```python
from build123d import *

# Parameters (mm, degrees)
F0_R     = 5
F1_DEPTH = 9
F2_R     = 3.5
F3_DEPTH = 8
F4_W     = 9.3990088471
F4_H     = 6
F5_DEPTH = 12.5
F7_DEPTH = 25
F8_R     = 1
F9_DEPTH = 8


with BuildPart() as f1:
    # F0 (on Front) → F1 (new body)
    with BuildSketch(Plane.XZ):
        Circle(F0_R)
    extrude(amount=F1_DEPTH)

    # F2 (on face) → F3 (join)
    with BuildSketch(Plane.XZ.offset(9)):
        Circle(F2_R)
    extrude(amount=F3_DEPTH)

    # F4 (on Right) → F5 (cut, symmetric)
    with BuildSketch(Plane.YZ):
        with Locations((-3.8004955764, 3)):
            Rectangle(F4_W, F4_H)
    extrude(amount=F5_DEPTH, both=True, mode=Mode.SUBTRACT)

    # F6 (on face) → F7 (cut)
    with BuildSketch(Plane(origin=(0, -8.5, 0), x_dir=(-1, 0, 0), z_dir=(0, 1, 0))):
        with BuildLine():
            Line((-1, 3), (1, 3))
            Line((1, 3), (1, 4.8989794856))
            ThreePointArc((1, 4.8989794856), (0, 5), (-1, 4.8989794856))
            Line((-1, 4.8989794856), (-1, 3))
        make_face()
    extrude(amount=-F7_DEPTH, mode=Mode.SUBTRACT)

    # F8 (on face) → F9 (join)
    with BuildSketch(Plane.XY):
        with Locations((0, -4)):
            Circle(F8_R)
    extrude(amount=F9_DEPTH)


solid = f1.part
```
Work out the finished part from the listing and answer in its coordinate system (mm). A direction names the side the tool comes from. Coordinates: 2 decimals unless noted, no trailing zeros. Loops run counter-clockwise (first coordinate to the right, second up) from the corner with the lowest first, then second, coordinate; pieces in that order, holes last. Notation, with made-up numbers: M 24.5,77.5 L 34.5,77.5 A22 cw 34.5,91.5 Z; hole C -27.5,68 d2. An arc over 180 degrees is marked long. Use CSV: the item, a comma, the result in double quotes. Start each with the question number.
(1) Find section C-C, the plane z = -1.75. Give the vertices of the cut face in (x, y), then the cut area to 3 significant figures.
(2) For faces 1 (the face through (-1, -11.79, 3.17)), 2 (the face through (0, -4, 8)), 3 (the face through (2.2, -9, -3.3)), determine the directions among +Z, -Z, +X, -X, +Y, -Y from which every point of the face is accessible in a straight line to the end or side of a thin tool.
(3) For a pull along X with two mould halves and no side action, classify faces 4 (the face through (1, -11.79, 3.18)), 5 (the face through (0, -3, 4)), 6 (the face through (0, -17, 0)) as +X half, -X half, draft (parallel to the pull), parting line (faces both ways), or undercut.
(4) Given pin 1 Ø1.5 at (x, z) = (-1.5, 2) entering from +Y; pin 2 Ø2 at (y, z) = (-9.5, -2) entering from -X; pin 3 Ø4 at (y, z) = (-2.5, 3) entering from +X, each flat-ended and moving along its own axis, determine where each tip first touches the part or whether it passes through.
(5) Find section B-B, the plane y = -4. Give the vertices of the cut face in (x, z).
(6) Find section A-A, the plane x = 0. Give the vertices of the cut face in (y, z).
(7) Consider line 1 (Y direction, x = 2.25, z = 4); line 2 (Y direction, x = -2.75, z = 1.75); line 3 (Z direction, x = -1.75, y = -6.5). Determine where each line is inside the solid, lowest interval first.
(8) Find section D-D, the plane x = -1.5. Give the vertices of the cut face in (y, z), then the cut area to 3 significant figures.
Recorded:
1,outline,"M -4.68,-9 L -3.03,-9 L -3.03,-17 L 3.03,-17 L 3.03,-9 L 4.68,-9 L 4.68,0 L -4.68,0 Z"
1,area,"133 mm^2"
2,face 1,"+Z, -Y"
2,face 2,"+Z, +X, -X, +Y, -Y"
2,face 3,"-Y"
3,face 4,"undercut"
3,face 5,"parting line"
3,face 6,"draft"
4,pin 1,"stops at y = -3.34"
4,pin 2,"stops at x = -4.87"
4,pin 3,"stops at x = 1"
5,outline,"M -5,0 A5 ccw 5,0 L 1,0 L 1,8 L -1,8 L -1,0 Z"
6,outline,"M -17,-3.5 L -9,-3.5 L -9,-5 L 0,-5 L 0,0 L -3,0 L -3,8 L -5,8 L -5,0 L -8.5,0 L -8.5,3 L -17,3 Z"
7,line 1,"y = -9 to -8.5"
7,line 2,"y = -17 to -8.5"
7,line 3,"z = -4.68 to 0"
8,outline,"M -17,-3.16 L -9,-3.16 L -9,-4.77 L 0,-4.77 L 0,0 L -8.5,0 L -8.5,4.77 L -9,4.77 L -9,3.16 L -17,3.16 Z"
8,area,"95.9 mm^2"
